Input: part model. Units: mm. Frame: model coordinates. Face numbers are marked on the shaded views. A direction names the side the tool comes from. Give positions to 0.01 mm unless a question says otherwise; leave off trailing zeros. Order: outer loops, then holes, each group sorted by start corner. A loop starts at its lowest first (then second) coordinate and runs counter-clockwise, first axis right, second up. Notation, with made-up numbers: M -27,11.5 L 25,11.5 A7 cw 25,22.5 Z; hole C 7.5,79 d5. An arc over 180 degrees is marked long. Use a Markdown table: item, result.
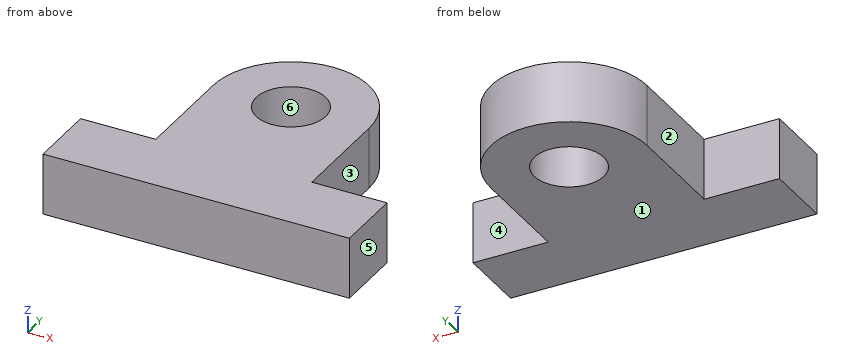
from build123d import *

# Parameters (mm, degrees)
SKETCH1_R           = 12.5
BOSS_EXTRUDE1_DEPTH = 11


with BuildPart() as part:
    # Sketch1 → Boss-Extrude1 (new, symmetric)
    with BuildSketch(Plane.XY):
        with BuildLine():
            Line((-55, 0), (55, 0))
            Line((55, 0), (55, 25))
            Line((55, 25), (28, 25))
            Line((28, 25), (28, 63))
            ThreePointArc((28, 63), (0, 91), (-28, 63))
            Line((-28, 63), (-28, 25))
            Line((-28, 25), (-55, 25))
            Line((-55, 25), (-55, 0))
        make_face()
        with Locations((0, 63)):
            Circle(SKETCH1_R, mode=Mode.SUBTRACT)
    extrude(amount=BOSS_EXTRUDE1_DEPTH, both=True)


solid = part.part
1) First-contact query: pin 1 Ø22.5 at (x, y) = (0, 63) entering from -Z; pin 2 Ø11 at (y, z) = (39.5, -1) entering from +X; pin 3 Ø4 at (x, z) = (18, 6.5) entering from +Y; pin 4 Ø4 at (x, z) = (40, 5) entering from -Y. Flat tips, straight axial feed; report the tip coordinate or a pass-through.
Response values:
| item | result |
|---|---|
| pin 1 | passes through |
| pin 2 | stops at x = 28 |
| pin 3 | stops at y = 85.98 |
| pin 4 | stops at y = 0 |
2) Cut plane A-A on x = 0. Return loops of the section in (y, z), and give its area (3 significant figures).
Response values:
| item | result |
|---|---|
| outline | M 0,-11 L 50.5,-11 L 50.5,11 L 0,11 Z; M 75.5,-11 L 91,-11 L 91,11 L 75.5,11 Z |
| area | 1,450 mm² |
3) Cut plane B-B on z = -8. Return loops of the section in (x, y), and give its area (3 significant figures).
Response values:
| item | result |
|---|---|
| outline | M -55,0 L 55,0 L 55,25 L 28,25 L 28,63 A28 ccw -28,63 L -28,25 L -55,25 Z; hole C 0,63 d25 |
| area | 5,620 mm² |
4) Material intervals for line 1 (Y direction, x = 0, z = -0.75); line 2 (Y direction, x = -45.5, z = -4.25); line 3 (X direction, y = 29.5, z = 6.75), sorted ascending. Write a range as from..to.
Response values:
| item | result |
|---|---|
| line 1 | y = 0..50.5, 75.5..91 |
| line 2 | y = 0..25 |
| line 3 | x = -28..28 |
5) Cut plane D-D on y = 35.5. Return loops of the section in (x, z), and give its area (3 significant figures).
Response values:
| item | result |
|---|---|
| outline | M -28,-11 L 28,-11 L 28,11 L -28,11 Z |
| area | 1,230 mm² |
6) Reachability of the marked faces 1, 2 and 3 from +Z, -Z, +X, -X, +Y, -Y: full face, straight path, thin tool, end or side. Return the list, or none.
Response values:
| item | result |
|---|---|
| face 1 | -Z, +X, -X, +Y, -Y |
| face 2 | +Z, -Z, -X, +Y |
| face 3 | +Z, -Z, +X, +Y |
7) Cut plane C-C on y = 68. Return loops of the section in (x, z).
Response values:
| item | result |
|---|---|
| outline | M -27.55,-11 L -11.46,-11 L -11.46,11 L -27.55,11 Z; M 11.46,-11 L 27.55,-11 L 27.55,11 L 11.46,11 Z |
8) Mould query, pull axis Y, two halves, no side actions, for the marked faces 4, 5 and 6. Classes: released by +Y, released by -Y, zero draft, split by the parting line, or undercut.
Response values:
| item | result |
|---|---|
| face 4 | released by +Y |
| face 5 | zero draft |
| face 6 | undercut |
